Study the drawing (mm; zero at the part's minimum x, y, z) and answer. Round coordinates to 2 decimals unless told otherwise and drop trailing zeros. Order: outer loops, then holes, each group sorted by start corner. A loop starts at its lowest first (then second) coordinate and runs counter-clockwise, first axis right, second up. Notation, with made-up numbers: (14, 52.5) - (72, 52.5) arc R19 cw to (72, 62.5) - close; hole circle Ø5 at (-10.75, 83.5). An arc over 180 degrees is marked (long way). Put each result on its own line as item: value.
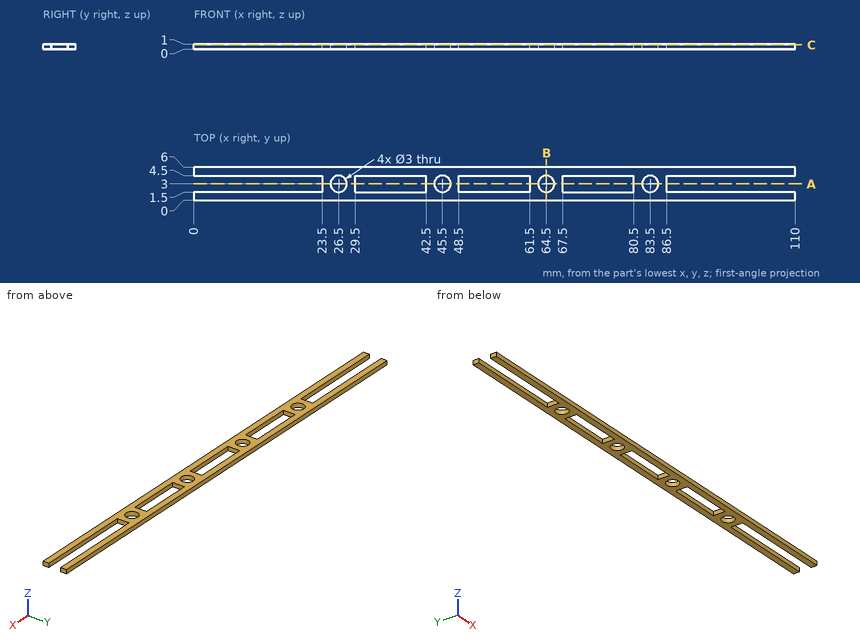
1) Given pin 1 Ø0.5 at (y, z) = (3.5, 0.5) entering from +X, flat-ended and moving along its own axis, determine where the tip first touches the part or whether it passes through.
Findings below:
pin 1: stops at x = 86.5
2) A cutting plane is placed at B-B on x = 64.5. Write down the section's boundary in (y, z), then the cut area to 3 significant figures.
Findings below:
outline: (0, 0) - (1.5, 0) - (1.5, 1) - (0, 1) - close; (4.5, 0) - (6, 0) - (6, 1) - (4.5, 1) - close
area: 3.00 mm2
3) A straight line is drawn through the part: L1, parallel to Y at x = 26.5, z = 0.35. Find the intervals that lie inside material, in ascending order. Write a range as from..to.
Findings below:
L1: y = 0..1.5, 4.5..6
4) A cutting plane is placed at C-C on z = 0.85. Write down the section's boundary in (x, y).
Findings below:
outline: (0, 0) - (110, 0) - (110, 1.5) - (86.5, 1.5) - (86.5, 4.5) - (110, 4.5) - (110, 6) - (0, 6) - (0, 4.5) - (23.5, 4.5) - (23.5, 1.5) - (0, 1.5) - close; hole circle Ø3 at (26.5, 3); hole (29.5, 1.5) - (42.5, 1.5) - (42.5, 4.5) - (29.5, 4.5) - close; hole circle Ø3 at (45.5, 3); hole (48.5, 1.5) - (61.5, 1.5) - (61.5, 4.5) - (48.5, 4.5) - close; hole circle Ø3 at (64.5, 3); hole (67.5, 1.5) - (80.5, 1.5) - (80.5, 4.5) - (67.5, 4.5) - close; hole circle Ø3 at (83.5, 3)
5) A cutting plane is placed at A-A on y = 3. Give the number of separate pieces and of enclosed holes in the cut face, then the cut area to 3 significant figures.
Findings below:
separate pieces: 8
enclosed holes: 0
area: 12.0 mm2
